The listing builds one solid part. Answer for the finished solid, in the listing's coordinates (mm). A direction names the side the tool comes from. Give positions to 0.01 mm unless a question says otherwise; leave off trailing zeros. Loops run counter-clockwise (first coordinate to the right, second up) from the corner with the lowest first, then second, coordinate; pieces in that order, holes last.
Item 1: Consider line 1 along Y through (x, z) = (9, 0.7); line 2 along X through (y, z) = (-1.15, 6.75); line 3 along Z through (x, y) = (7.25, -2.25). Determine where each line is inside the solid, lowest interval first.
Item 2: Section A-A, the plane y = 0 is taken. Give the vertices of the cut face in (x, z), and give its area (3 significant figures).
Item 3: Each of these flat-tipped pins is pushed along its axis until it touches: pin 1 Ø3 at (y, z) = (-0.5, 7.5) entering from +X; pin 2 Ø1.6 at (x, y) = (0.5, 0) entering from +Z; pin 3 Ø2 at (x, y) = (6.5, 0.5) entering from -Z. Where does it stop, or does it pass through?
Item 4: The mould has two halves that part along X. Classify faces 4 (the face through (-6, 0, 5)), 5 (the face through (-4, 0, 11)), 6 (the face through (3, 0, 0)): pulls with the +X half, pulls with the -X half, needs draft (parallel to the pull), parting line crosses it, or undercut.
Item 5: Section B-B, the plane x = 9 is taken. Give the vertices of the cut face in (y, z), and give its area (3 significant figures).
Item 6: Section C-C, the plane z = 4.25 is taken. Give the vertices of the cut face in (x, y), and give its area (3 significant figures).
Item 7: Section D-D, the plane z = -8.5 is taken. Give the vertices of the cut face in (x, y).
Item 8: A tool of negligible diameter and unlimited length cuts with its end or side. For faces 1 (the face through (4.746, -0.585, -4.93)), 2 (the face through (1.6, 0, 6)), 3 (the face through (2, 3, 5)), from which of +Z, -Z, +X, -X, +Y, -Y can it reach the whole face along a straight path? Write none if from no direction.
from build123d import *

# Parameters (mm, degrees)
F1_DEPTH = 2
F2_W     = 4.4
F2_H     = 6
F3_DEPTH = 9
F4_R     = 0.75
F5_DEPTH = 10
F6_R     = 1.75
F7_DEPTH = 12.001


with BuildPart() as f1:
    # F0 (on Top) → F1 (new body)
    with BuildSketch(Plane.XY):
        with BuildLine():
            Line((6, 3), (-6, 3))
            Line((-6, 3), (-6, -3))
            Line((-6, -3), (6, -3))
            Line((6, -3), (9.6, -3))
            ThreePointArc((9.6, -3), (12.6, 0), (9.6, 3))
            Line((9.6, 3), (6, 3))
        make_face()
    extrude(amount=F1_DEPTH)

    # F2 (on face) → F3 (join)
    with BuildSketch(Plane.XY.offset(2)):
        with Locations((-3.8, 0)):
            Rectangle(F2_W, F2_H)
        with Locations((3.8, 0)):
            Rectangle(F2_W, F2_H)
    extrude(amount=F3_DEPTH)

    # F4 (on face) → F5 (join)
    with BuildSketch(Plane(origin=(0, 0, 0), x_dir=(1, 0, 0), z_dir=(0, 0, -1))):
        with Locations((-4.4, 1.25)):
            Circle(F4_R)
        with Locations((4.4, 1.25)):
            Circle(F4_R)
        with Locations((4.4, -1.25)):
            Circle(F4_R)
        with Locations((-4.4, -1.25)):
            Circle(F4_R)
    extrude(amount=F5_DEPTH)

    # F6 (on face) → F7 (cut, through all)
    with BuildSketch(Plane.XY.offset(2)):
        with Locations((9, 0)):
            Circle(F6_R)
    extrude(amount=-F7_DEPTH, mode=Mode.SUBTRACT)


solid = f1.part
Worked answers:
1. line 1: y = -3 to -1.75, 1.75 to 3
1. line 2: x = -6 to -1.6, 1.6 to 6
1. line 3: z = 0 to 2
2. outline: (-6, 0) - (7.25, 0) - (7.25, 2) - (6, 2) - (6, 11) - (1.6, 11) - (1.6, 2) - (-1.6, 2) - (-1.6, 11) - (-6, 11) - close; (10.75, 0) - (12.6, 0) - (12.6, 2) - (10.75, 2) - close
2. area: 109 mm2
3. pin 1: stops at x = 6
3. pin 2: stops at z = 2
3. pin 3: stops at z = 0
4. face 4: pulls with the -X half
4. face 5: needs draft
4. face 6: undercut
5. outline: (-3, 0) - (-1.75, 0) - (-1.75, 2) - (-3, 2) - close; (1.75, 0) - (3, 0) - (3, 2) - (1.75, 2) - close
5. area: 5.00 mm2
6. outline: (-6, -3) - (-1.6, -3) - (-1.6, 3) - (-6, 3) - close; (1.6, -3) - (6, -3) - (6, 3) - (1.6, 3) - close
6. area: 52.8 mm2
7. outline: circle Ø1.5 at (-4.4, -1.25); circle Ø1.5 at (-4.4, 1.25); circle Ø1.5 at (4.4, -1.25); circle Ø1.5 at (4.4, 1.25)
8. face 1: -Z
8. face 2: +Z, +Y, -Y
8. face 3: +Z, -Z, +X, -X, +Y
